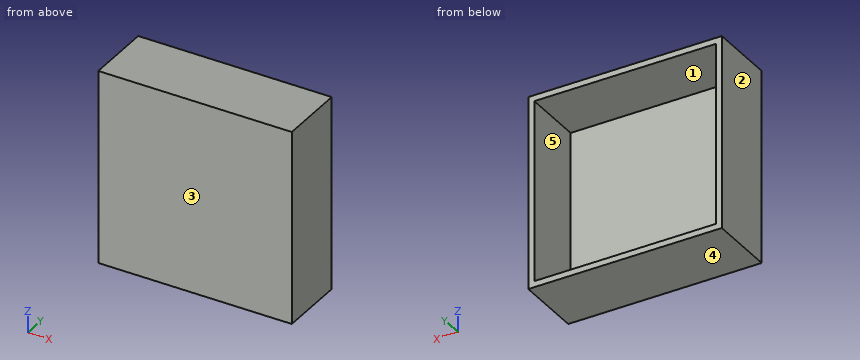
from build123d import *

# Parameters (mm, degrees)
ESQUISSE1_W        = 150
ESQUISSE1_H        = 150
BOSS_EXTRU_1_DEPTH = 50
COQUE2_T           = 5


with BuildPart() as part:
    # Esquisse1 → Boss.-Extru.1 (new body)
    with BuildSketch(Plane(origin=(0, 0, 0), x_dir=(1, 0, 0), z_dir=(0, 1, 0))):
        Rectangle(ESQUISSE1_W, ESQUISSE1_H)
    extrude(amount=BOSS_EXTRU_1_DEPTH)

    # Coque2
    coque2_openings = [part.faces().sort_by_distance(p)[0] for p in [
        (0, 50, 0),
    ]]
    offset(amount=COQUE2_T, openings=coque2_openings, kind=Kind.INTERSECTION)


solid = part.part
Read the model definition and answer for the solid it produces. Units are mm, in the model's axes. Face numbers are marked on the shaded views. A direction names the side the tool comes from. Round coordinates to 2 decimals unless told otherwise and drop trailing zeros. Loops run counter-clockwise (first coordinate to the right, second up) from the corner with the lowest first, then second, coordinate; pieces in that order, holes last.
Q1. This flat-tipped pin is pushed along its axis until it touches: pin 1 (4 mm diameter, centred on x = -24, z = 20.5, fed in from +Y). Where does it stop, or does it pass through?
Q2. Determine the mould class of the marked faces 1, 2 and 3 for opening direction X: released by +X, released by -X, zero draft, split by the parting line, or undercut.
Q3. Section B-B on z = 26 is taken. Write down the section's boundary in (x, y), and give its area (3 significant figures).
Q4. Consider probe 1 along Z at (x, y) = (-11, 19.5); probe 2 along Y at (x, z) = (62, 44.5). Determine where each line is inside the solid, lowest interval first.
Q5. Section A-A on y = 40.5 is taken. Write down the section's boundary in (x, z), and give its area (3 significant figures).
Q6. Which of the six approach directions +Z, -Z, +X, -X, +Y, -Y give full straight-line access (tool end or side, diameter ignored) to the marked faces 4 and 5?
Q7. Section C-C on x = -31.5 is taken. Write down the section's boundary in (y, z), and give its area (3 significant figures).
Output:
1. pin 1: stops at y = 0
2. face 1: undercut
2. face 2: released by -X
2. face 3: zero draft
3. outline: (-80, -5) - (80, -5) - (80, 50) - (75, 50) - (75, 0) - (-75, 0) - (-75, 50) - (-80, 50) - close
3. area: 1,300 mm2
4. probe 1: z = -80 to -75, 75 to 80
4. probe 2: y = -5 to 0
5. outline: (-80, -80) - (80, -80) - (80, 80) - (-80, 80) - close; hole (-75, -75) - (75, -75) - (75, 75) - (-75, 75) - close
5. area: 3,100 mm2
6. face 4: -Z, +X, -X, +Y, -Y
6. face 5: +Y
7. outline: (-5, -80) - (50, -80) - (50, -75) - (0, -75) - (0, 75) - (50, 75) - (50, 80) - (-5, 80) - close
7. area: 1,300 mm2
